Autodesk Inventor part; units mm, degrees
ref_plane "YZ Plane" through (0, 0, 0) normal (1, 0, 0) x (0, 1, 0)
ref_plane "XZ Plane" through (0, 0, 0) normal (0, 1, 0) x (-1, 0, 0)
ref_plane "XY Plane" through (0, 0, 0) normal (0, 0, 1) x (1, 0, 0)
sketch "Sketch1" plane through (0, 0, 0) normal (0, 0, 1) x (1, 0, 0)
  line L0 (-40, 25) -> (40, 25)
  line L1 (40, 25) -> (40, -25)
  line L2 (40, -25) -> (-40, -25)
  line L3 (-40, -25) -> (-40, 25)
  line L4 (-40, 25) -> (40, -25) construction
  line L5 (40, 25) -> (-40, -25) construction
  point P0 (0, 0)
  dimension "d0" = 80
  dimension "d1" = 50
extrude "Extrusion1" add sketch "Sketch1" along normal blind 5
sketch "Sketch2" plane through (0, 0, 0) normal (0, 0, 1) x (1, 0, 0)
  line L0 (0, 0) -> (-30, 0) construction
  line L1 (0, 0) -> (30, 0) construction
  circle A0 centre (-30, 0) radius 3.75
  circle A1 centre (30, 0) radius 3.75
  dimension "d4" = 30
  dimension "d5" = 30
  dimension "d6" = 7.5
  dimension "d7" = 7.5
extrude "Extrusion2" cut sketch "Sketch2" along normal through all
sketch "Sketch3" plane through (0, 0, 0) normal (0, 0, 1) x (1, 0, 0)
  line L0 (-25, 25) -> (25, 25)
  line L1 (25, 25) -> (25, -25)
  line L2 (25, -25) -> (-25, -25)
  line L3 (-25, -25) -> (-25, 25)
  line L4 (-25, 25) -> (25, -25) construction
  line L5 (25, 25) -> (-25, -25) construction
  point P0 (0, 0)
  dimension "d10" = 50
  dimension "d11" = 50
extrude "Extrusion3" add sketch "Sketch3" along normal blind 25
sketch "Sketch4" plane through (0, 0, 25) normal (0, 0, 1) x (1, 0, 0)
  circle A0 centre (0, 0) radius 12.5
  dimension "d14" = 25
extrude "Extrusion4" add sketch "Sketch4" along normal blind 90
sketch "Sketch5" plane through (0, 0, 115) normal (0, 0, 1) x (1, 0, 0)
  circle A0 centre (0, 0) radius 16.25 construction
  line L0 (16.25, 0) -> (8.125, -14.0729)
  line L1 (8.125, -14.0729) -> (-8.125, -14.0729)
  line L2 (-8.125, -14.0729) -> (-16.25, 0)
  line L3 (-16.25, 0) -> (-8.125, 14.0729)
  line L4 (-8.125, 14.0729) -> (8.125, 14.0729)
  line L5 (8.125, 14.0729) -> (16.25, 0)
  dimension "d17" = 32.5
extrude "Extrusion5" add sketch "Sketch5" along normal blind 5
chamfer "Chamfer1" distance 5 angle 45 4 edges at (40, -25, 2.5) (40, 25, 2.5) (-40, -25, 2.5) (-40, 25, 2.5)
properties part number "UpperArm"
Geometry check sheet. Reference: the model listing, model coordinates, mm. A direction names the side the tool comes from. Give positions to 0.01 mm unless a question says otherwise; leave off trailing zeros. Order: outer loops, then holes, each group sorted by start corner. A loop starts at its lowest first (then second) coordinate and runs counter-clockwise, first axis right, second up.
1. Sectioned sample at A-A (x = 30). Record the boundary of the cut face in (y, z).
Completed:
outline: (-25, 0) - (-3.75, 0) - (-3.75, 5) - (-25, 5) - close; (3.75, 0) - (25, 0) - (25, 5) - (3.75, 5) - close
2. Draft check along X on faces 6 (the face through (0, 25, 12)), 7 (the face through (-38, 22, 3)), 8 (the face through (-33.746, -0.165, 2.465)). Enter one of: pulls with the +X half, pulls with the -X half, needs draft (parallel to the pull), parting line crosses it, or undercut.
Completed:
face 6: needs draft
face 7: pulls with the -X half
face 8: undercut
3. Sectioned sample at D-D (z = 97). Record the boundary of the cut face in (x, y).
Completed:
outline: circle Ø25 at (0, 0)
4. Depth check by flat-ended pin: pin 1 (16.5 mm diameter, centred on x = -36, y = -5, fed in from +Z); pin 2 (5.5 mm diameter, centred on x = -3, z = 117, fed in from -Y); pin 3 (8 mm diameter, centred on y = 8, z = 22, fed in from +X). Enter the tip coordinate at first touch or a pass-through.
Completed:
pin 1: stops at z = 5
pin 2: stops at y = -14.07
pin 3: stops at x = 25
5. Access from +Z, -Z, +X, -X, +Y, -Y to the whole of each face (thin tool, end or side, straight path). Record for faces 1 (the face through (11.923, -3.755, 69.37)), 2 (the face through (-12.244, 6.938, 117.465)), 3 (the face through (25, 0, 15)), 4 (the face through (-12.131, -7.135, 117.465)), 5 (the face through (0, -14.073, 117)).
Completed:
face 1: none
face 2: +Z, -X, +Y
face 3: +Z, +X, +Y, -Y
face 4: +Z, -X, -Y
face 5: +Z, +X, -X, -Y
6. Sectioned sample at B-B (y = 5). Record the boundary of the cut face in (x, z), then the cut area to 3 significant figures.
Completed:
outline: (-40, 0) - (40, 0) - (40, 5) - (25, 5) - (25, 25) - (11.46, 25) - (11.46, 115) - (13.36, 115) - (13.36, 120) - (-13.36, 120) - (-13.36, 115) - (-11.46, 115) - (-11.46, 25) - (-25, 25) - (-25, 5) - (-40, 5) - close
area: 3,600 mm2
7. Scan lines: line 1 (X direction, y = 0, z = 1.4); line 2 (Y direction, x = -30, z = 1.95); line 3 (Z direction, x = -12.5, y = -2.5). Record each from-to range of solid material in increasing order.
Completed:
line 1: x = -40 to -33.75, -26.25 to 26.25, 33.75 to 40
line 2: y = -25 to -3.75, 3.75 to 25
line 3: z = 0 to 25, 115 to 120
8. Sectioned sample at C-C (x = -5). Record the boundary of the cut face in (y, z), then the cut area to 3 significant figures.
Completed:
outline: (-25, 0) - (25, 0) - (25, 25) - (11.46, 25) - (11.46, 115) - (14.07, 115) - (14.07, 120) - (-14.07, 120) - (-14.07, 115) - (-11.46, 115) - (-11.46, 25) - (-25, 25) - close
area: 3,450 mm2
